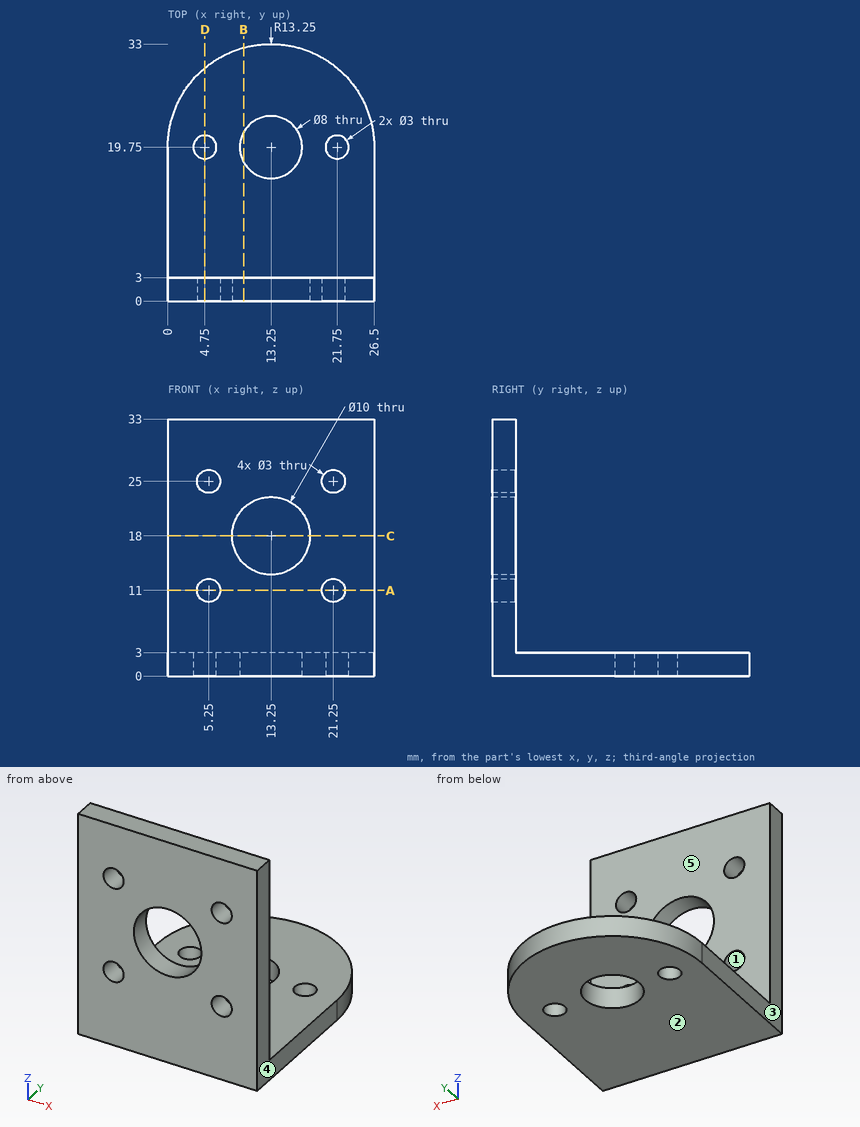
For this review, use the dimensioned drawing (mm, ordinates from the lowest corner) and the shaded views. A direction names the side the tool comes from. Give positions to 0.01 mm unless a question says otherwise; leave off trailing zeros. Order: outer loops, then holes, each group sorted by start corner. A loop starts at its lowest first (then second) coordinate and runs counter-clockwise, first axis right, second up. Notation, with made-up numbers: (65.5, 41) - (107.5, 41) arc R16 cw to (107.5, 49) - close; hole circle Ø5 at (-35.75, 11). An arc over 180 degrees is marked (long way). Write item = value, one per line. Start each with the question number.
Q1. We need section C-C on z = 18. State the section outline as (x, y) points, plus the area to 3 significant figures.
Q2. We need section B-B on x = 9.75. State the section outline as (y, z) points.
Q3. To check wall thickness, follow L1, parallel to X at y = 1, z = 25; L2, parallel to X at y = 1.15, z = 18; L3, parallel to Y at x = 21.75, z = 20. State the ranges of each line that lie inside material, in increasing order. Write a range as from..to.
Q4. Tool access review of the marked faces 4 and 5: name each direction out of +Z, -Z, +X, -X, +Y, -Y from which nothing blocks a thin tool from reaching the whole face with its end or side.
Q5. Mouldability with a two-part tool opening along Z and no side actions: class the marked faces 1, 2 and 3 as released by +Z, released by -Z, zero draft, split by the parting line, or undercut.
Q6. Clearance check with flat-ended pins moving along their axes: pin 1 Ø2.5 at (x, z) = (5.25, 11) entering from -Y; pin 2 Ø13 at (x, z) = (12.5, 21) entering from +Y; pin 3 Ø5 at (x, y) = (3, 29) entering from +Z. State where each tip first meets the part, or that it passes through.
Q7. We need section D-D on x = 4.75. State the section outline as (y, z) points, plus the area to 3 significant figures.
Q8. We need section A-A on z = 11. State the section outline as (x, y) points, plus the area to 3 significant figures.
Working result:
q1.outline = (0, 0) - (8.25, 0) - (8.25, 3) - (0, 3) - close; (18.25, 0) - (26.5, 0) - (26.5, 3) - (18.25, 3) - close
q1.area = 49.5 mm²
q2.outline = (0, 0) - (17.81, 0) - (17.81, 3) - (3, 3) - (3, 14.43) - (0, 14.43) - close; (0, 21.57) - (3, 21.57) - (3, 33) - (0, 33) - close; (21.69, 0) - (32.53, 0) - (32.53, 3) - (21.69, 3) - close
q3.L1 = 0..3.75, 6.75..19.75, 22.75..26.5
q3.L2 = 0..8.25, 18.25..26.5
q3.L3 = 0..3
q4.face_4 = +Z, -Z, +X, +Y, -Y
q4.face_5 = +Z, +X, -X, +Y
q5.face_1 = undercut
q5.face_2 = released by -Z
q5.face_3 = zero draft
q6.pin_1 = through
q6.pin_2 = 3
q6.pin_3 = 3
q7.outline = (0, 0) - (18.25, 0) - (18.25, 3) - (3, 3) - (3, 9.59) - (0, 9.59) - close; (0, 12.41) - (3, 12.41) - (3, 23.59) - (0, 23.59) - close; (0, 26.41) - (3, 26.41) - (3, 33) - (0, 33) - close; (21.25, 0) - (29.91, 0) - (29.91, 3) - (21.25, 3) - close
q7.area = 154 mm²
q8.outline = (0, 0) - (3.75, 0) - (3.75, 3) - (0, 3) - close; (6.75, 0) - (19.75, 0) - (19.75, 3) - (6.75, 3) - close; (22.75, 0) - (26.5, 0) - (26.5, 3) - (22.75, 3) - close
q8.area = 61.5 mm²
